Model file for the job. Use its own axes, mm. Round coordinates to 2 decimals unless told otherwise and drop trailing zeros. Order: outer loops, then holes, each group sorted by start corner. A loop starts at its lowest first (then second) coordinate and runs counter-clockwise, first axis right, second up. Notation, with made-up numbers: M 22.25,-36.75 L 78.25,-36.75 A27 ccw 78.25,-16.75 Z; hole C 65,42.25 d4. An arc over 180 degrees is marked long. Return JSON: item names as keys, results as strings. Group by question number.
Item 1: Pin check, flat tips, straight feed: pin 1 Ø6 at (x, z) = (-22.5, -117.5) entering from -Y; pin 2 Ø6 at (x, z) = (-100.5, -50) entering from -Y. Stop position of each tip, or through.
Item 2: Probe line 1 along X through (y, z) = (0.6, -98); line 2 along Z through (x, y) = (-102.5, 0.8); line 3 along Z through (x, y) = (-27, 1.4). List the from-to ranges inside material, lowest first.
Item 3: Slice it at B-B on x = -22.5. Write the cut outline in (y, z), then the cut area to 3 significant figures.
Item 4: Pull direction Z, two halves, no side cores. Call faces 1 (the face through (-124, 1, -2)), 2 (the face through (-123, 1, -129)), 3 (the face through (-21.42, 0.99, -12.62)): pulls with the +Z half, pulls with the -Z half, needs draft (parallel to the pull), parting line crosses it, or undercut.
Item 5: Slice it at A-A on z = -24. Write the cut outline in (x, y), then the cut area to 3 significant figures.
Item 6: Slice it at C-C on y = 0.45. Give the number of separate pieces and of enclosed holes in the cut face, then the cut area to 3 significant figures.
Autodesk Inventor part; units mm, degrees
ref_plane "YZ Plane" through (0, 0, 0) normal (1, 0, 0) x (0, 1, 0)
ref_plane "XZ Plane" through (0, 0, 0) normal (0, 1, 0) x (-1, 0, 0)
ref_plane "XY Plane" through (0, 0, 0) normal (0, 0, 1) x (1, 0, 0)
sketch "Sketch1" plane through (0, 0, 0) normal (0, 1, 0) x (-1, 0, 0)
  line L0 (0, 0) -> (125, 0)
  line L1 (125, 0) -> (125, -130)
  line L2 (125, -130) -> (0, -130)
  line L3 (0, -130) -> (0, 0)
  circle A0 centre (102.5, -17.5) radius 5
  circle A1 centre (102.5, -117.5) radius 5
  circle A2 centre (22.5, -17.5) radius 5
  circle A3 centre (22.5, -117.5) radius 5
  dimension "d0" = 130
  dimension "d1" = 125
  dimension "d2" = 10
  dimension "d3" = 10
  dimension "d4" = 100
  dimension "d5" = 10
  dimension "d6" = 10
  dimension "d7" = 100
  dimension "d8" = 80
  dimension "d9" = 80
  dimension "d10" = 17.5
  dimension "d11" = 22.5
  dimension "d12" = 17.5
  dimension "d13" = 22.5
extrude "Extrusion1" add sketch "Sketch1" along normal blind 2
sketch "Sketch2" plane through (0, 2, 0) normal (0, 1, 0) x (1, 0, 0)
  line L0 (-90, 115.6784) -> (-35, 115.6784) construction
  line L1 (-35, 115.6784) -> (-35, 15.6784) construction
  line L2 (-35, 15.6784) -> (-90, 15.6784) construction
  line L3 (-90, 15.6784) -> (-90, 115.6784) construction
  line L4 (0, 130) -> (-125, 130)
  line L5 (-125, 130) -> (-125, 0)
  line L6 (-125, 0) -> (0, 0)
  line L7 (0, 0) -> (0, 130)
  circle A0 centre (-22.5, 117.5) radius 5
  circle A1 centre (-22.5, 17.5) radius 5
  circle A2 centre (-102.5, 117.5) radius 5
  circle A3 centre (-102.5, 17.5) radius 5
  line L8 (-35, 40.5) -> (-33, 40.5)
  line L9 (-33, 40.5) -> (-33, 19.5)
  line L10 (-33, 19.5) -> (-35, 19.5)
  line L11 (-35, 19.5) -> (-35, 40.5)
  line L12 (-35, 110.5) -> (-33, 110.5)
  line L13 (-33, 110.5) -> (-33, 89.5)
  line L14 (-33, 89.5) -> (-35, 89.5)
  line L15 (-35, 89.5) -> (-35, 110.5)
  line L16 (-90, 110.5) -> (-92, 110.5)
  line L17 (-92, 110.5) -> (-92, 89.5)
  line L18 (-92, 89.5) -> (-90, 89.5)
  line L19 (-90, 89.5) -> (-90, 110.5)
  line L20 (-90, 40.5) -> (-92, 40.5)
  line L21 (-92, 40.5) -> (-92, 19.5)
  line L22 (-92, 19.5) -> (-90, 19.5)
  line L23 (-90, 19.5) -> (-90, 40.5)
  dimension "d16" = 55
  dimension "d17" = 100
  dimension "d18" = 125
  dimension "d19" = 35
  dimension "d20" = 2
  dimension "d21" = 2
  dimension "d22" = 2
  dimension "d23" = 2
  dimension "d24" = 21
  dimension "d25" = 21
  dimension "d26" = 21
  dimension "d27" = 21
  dimension "d28" = 19.5
  dimension "d29" = 19.5
  dimension "d30" = 19.5
  dimension "d31" = 19.5
extrude "Extrusion2" cut sketch "Sketch2" against normal through all contours L8 L9 L10 L11 | L12 L13 L14 L15 | L19 L18 L17 L16 | L23 L22 L21 L20
fillet "Fillet1" radius 5 4 edges at (0, 1, 0) (0, 1, -130) (-125, 1, 0) (-125, 1, -130)
equation "\"d19\" = -0.5 * d16 + 0.5 * d18"
equation "\"d25\" = d24"
equation "\"d26\" = d27"
equation "\"d27\" = d25"
equation "\"d29\" = d28"
equation "\"d30\" = d29"
equation "\"d31\" = d28"
properties part number "plade_til_beslag"
Output values:
{
 "1": {"pin 1": "through", "pin 2": "y = 0"},
 "2": {"line 1": "-125 to -92, -90 to -35, -33 to 0", "line 2": "-130 to -122.5, -112.5 to -22.5, -12.5 to 0", "line 3": "-130 to -119.68, -115.32 to -19.68, -15.32 to 0"},
 "3": {"outline": "M 0,-130 L 2,-130 L 2,-122.5 L 0,-122.5 Z; M 0,-112.5 L 2,-112.5 L 2,-22.5 L 0,-22.5 Z; M 0,-12.5 L 2,-12.5 L 2,0 L 0,0 Z", "area": "220 mm²"},
 "4": {"face 1": "pulls with the +Z half", "face 2": "pulls with the -Z half", "face 3": "undercut"},
 "5": {"outline": "M -125,0 L -92,0 L -92,2 L -125,2 Z; M -90,0 L -35,0 L -35,2 L -90,2 Z; M -33,0 L 0,0 L 0,2 L -33,2 Z", "area": "242 mm²"},
 "6": {"separate pieces": "1", "enclosed holes": "8", "area": "15,700 mm²"}
}
